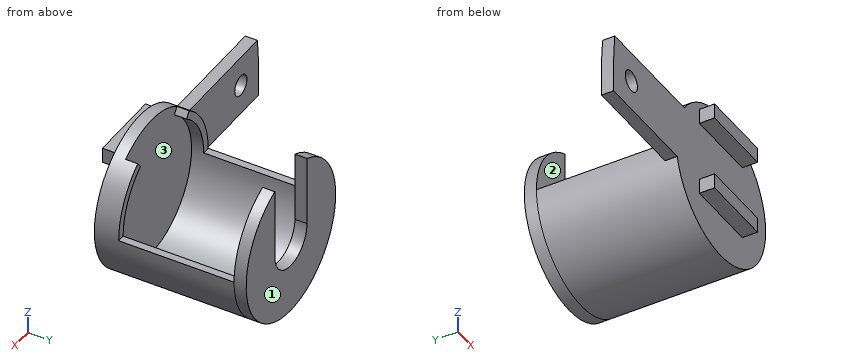
from build123d import *

# Parameters (mm, degrees)
CROQUIS1_R              = 12.5
CROQUIS1_R_2            = 11.25
SALIENTE_EXTRUIR1_DEPTH = 21
CORTAR_EXTRUIR1_DEPTH   = 19
CROQUIS3_R              = 12.5
SALIENTE_EXTRUIR2_DEPTH = 2
SALIENTE_EXTRUIR3_DEPTH = 2
CORTAR_EXTRUIR2_DEPTH   = 2
CROQUIS6_R              = 1.7
SALIENTE_EXTRUIR4_DEPTH = 2
CROQUIS8_W              = 12
CROQUIS8_H              = 2.5
SALIENTE_EXTRUIR5_DEPTH = 2.5


with BuildPart() as part:
    # Croquis1 → Saliente-Extruir1 (new body)
    with BuildSketch(Plane(origin=(0, 0, 0), x_dir=(1, 0, 0), z_dir=(0, 1, 0))):
        Circle(CROQUIS1_R)
        Circle(CROQUIS1_R_2, mode=Mode.SUBTRACT)
    extrude(amount=SALIENTE_EXTRUIR1_DEPTH)

    # Croquis2 → Cortar-Extruir1 (cut)
    with BuildSketch(Plane(origin=(0, 21, 0), x_dir=(1, 0, 0), z_dir=(0, 1, 0))):
        with BuildLine():
            Line((-12.5, 0), (12.5, 0))
            ThreePointArc((12.5, 0), (0, -12.5), (-12.5, 0))
        make_face()
    extrude(amount=-CORTAR_EXTRUIR1_DEPTH, mode=Mode.SUBTRACT)

    # Croquis3 → Saliente-Extruir2 (add)
    with BuildSketch(Plane.XZ):
        Circle(CROQUIS3_R)
    extrude(amount=SALIENTE_EXTRUIR2_DEPTH)

    # Croquis4 → Saliente-Extruir3 (add)
    with BuildSketch(Plane(origin=(0, 21, 0), x_dir=(1, 0, 0), z_dir=(0, 1, 0))):
        with BuildLine():
            Line((-4.5, 0), (-4.5, -11.66190379))
            ThreePointArc((-4.5, -11.66190379), (0, 12.5), (4.5, -11.66190379))
            Line((4.5, -11.66190379), (4.5, 0))
            ThreePointArc((4.5, 0), (0, 4.5), (-4.5, 0))
        make_face()
    extrude(amount=SALIENTE_EXTRUIR3_DEPTH)

    # Croquis5 → Cortar-Extruir2 (cut)
    with BuildSketch(Plane(origin=(0, 2, 0), x_dir=(1, 0, 0), z_dir=(0, 1, 0))):
        with BuildLine():
            Line((0, 0), (-7.169705454, -10.239400554))
            ThreePointArc((-7.169705454, -10.239400554), (0, -12.5), (7.169705454, -10.239400554))
            Line((7.169705454, -10.239400554), (0, 0))
        make_face()
    extrude(amount=-CORTAR_EXTRUIR2_DEPTH, mode=Mode.SUBTRACT)

    # Croquis6 → Saliente-Extruir4 (add)
    with BuildSketch(Plane(origin=(0, 0, 0), x_dir=(1, 0, 0), z_dir=(0, 1, 0))):
        with BuildLine():
            Line((-29.628729703, -7.2), (-10.218121158, -7.2))
            ThreePointArc((-10.218121158, -7.2), (-12.265620132, -2.409266026), (-12.182364303, 2.8))
            Line((-12.182364303, 2.8), (-29.943977582, 2.8))
            ThreePointArc((-29.943977582, 2.8), (-29.965242476, -2.205639433), (-29.628729703, -7.2))
        make_face()
        with Locations((-25, -2.2)):
            Circle(CROQUIS6_R, mode=Mode.SUBTRACT)
    extrude(amount=-SALIENTE_EXTRUIR4_DEPTH)

    # Croquis8 → Saliente-Extruir5 (add)
    with BuildSketch(Plane.XZ.offset(2)):
        with Locations((0, 8.45)):
            Rectangle(CROQUIS8_W, CROQUIS8_H)
        with Locations((0, -4.05)):
            Rectangle(CROQUIS8_W, CROQUIS8_H)
    extrude(amount=SALIENTE_EXTRUIR5_DEPTH)


solid = part.part
The listing builds one solid part. Answer for the finished solid, in the listing's coordinates (mm). Face numbers are marked on the shaded views. Give positions to 0.01 mm unless a question says otherwise; leave off trailing zeros. Write each loop counter-clockwise with the first axis right and the second up, starting at its lowest first coordinate (ties: lowest second). Pieces come first, ordered by that corner, then holes. Notation, with made-up numbers: (17, -29) -> (39, -29) arc R22 ccw to (39, -20) -> close; hole circle Ø1 at (67, 86). An arc over 180 degrees is marked (long way). Use a Markdown table: item, result.
(1) Section D-D, the plane z = 6.25 is taken. Determine the outline of the cut face in (x, y), then the cut area to 3 significant figures.
Return value:
| item | result |
|---|---|
| outline | (-29.72, -2) -> (10.83, -2) -> (10.83, 2) -> (9.35, 2) -> (9.35, 0) -> (-9.35, 0) -> (-9.35, 2) -> (-10.83, 2) -> (-10.83, 0) -> (-29.72, 0) -> close; (-10.83, 21) -> (-4.5, 21) -> (-4.5, 23) -> (-10.83, 23) -> close; (4.5, 21) -> (10.83, 21) -> (10.83, 23) -> (4.5, 23) -> close |
| area | 112 mm2 |
(2) Section A-A, the plane x = -25 is taken. Determine the outline of the cut face in (y, z).
Return value:
| item | result |
|---|---|
| outline | (-2, -2.8) -> (0, -2.8) -> (0, 0.5) -> (-2, 0.5) -> close; (-2, 3.9) -> (0, 3.9) -> (0, 7.2) -> (-2, 7.2) -> close |
(3) Section B-B, the plane z = 2.2 is taken. Determine the outline of the cut face in (x, y), then the cut area to 3 significant figures.
Return value:
| item | result |
|---|---|
| outline | (-29.97, -2) -> (-26.7, -2) -> (-26.7, 0) -> (-29.97, 0) -> close; (-23.3, -2) -> (12.3, -2) -> (12.3, 2) -> (11.03, 2) -> (11.03, 0) -> (-11.03, 0) -> (-11.03, 2) -> (-12.3, 2) -> (-12.3, 0) -> (-23.3, 0) -> close; (-12.3, 21) -> (-4.5, 21) -> (-4.5, 23) -> (-12.3, 23) -> close; (4.5, 21) -> (12.3, 21) -> (12.3, 23) -> (4.5, 23) -> close |
| area | 114 mm2 |
(4) Section C-C, the plane y = -0.5 is taken. Determine the outline of the cut face in (x, z), then the cut area to 3 significant figures.
Return value:
| item | result |
|---|---|
| outline | (-29.94, -2.8) -> (-12.18, -2.8) arc R12.5 ccw (long way) to (-10.22, 7.2) -> (-29.63, 7.2) arc R70 ccw to start; hole circle Ø3.4 at (-25, 2.2) |
| area | 661 mm2 |
(5) Find the intervals of material crossed by probe 1 along Y at (x, z) = (-10.5, 6.5); probe 2 along Y at (x, z) = (-2, -4.75); probe 3 along Z at (x, y) = (0, 16), in increasing order. Write a range as from..to.
Return value:
| item | result |
|---|---|
| probe 1 | -2..2, 21..23 |
| probe 2 | -4.5..0, 21..23 |
| probe 3 | -12.5..-11.25 |
(6) Flat-ended cylindrical pins translate along their axes: P1, Ø1, axis at y = 21.5, z = 3.5, coming from the +X side; P2, Ø0.6, axis at y = 22, z = 6, coming from the -X side; P3, Ø0.8, axis at y = -2.5, z = -4, coming from the +X side; P4, Ø4, axis at x = 1, z = 10, coming from the -Y side. Find the tip coordinate at first contact, or state that the pin passes through.
Return value:
| item | result |
|---|---|
| P1 | x = 12.13 |
| P2 | x = -11.12 |
| P3 | x = 6 |
| P4 | y = -4.5 |
(7) Determine the mould class of the marked faces 1, 2 and 3 for opening direction Y: released by +Y, released by -Y, zero draft, split by the parting line, or undercut.
Return value:
| item | result |
|---|---|
| face 1 | released by +Y |
| face 2 | undercut |
| face 3 | undercut |
